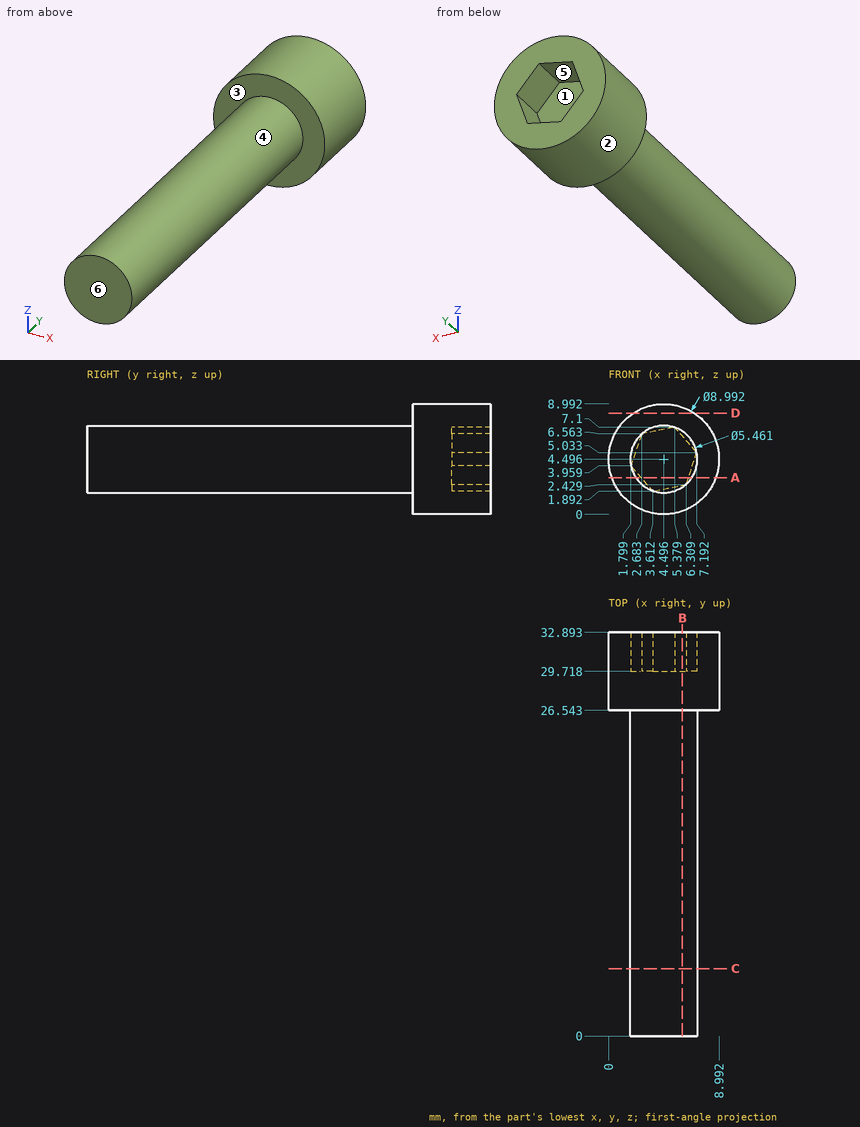
The drawing under review shows one solid part. Ordinate dimensions are in mm from its lowest x, y, z. A direction names the side the tool comes from. Coordinates: 2 decimals unless noted, no trailing zeros. Loops run counter-clockwise (first coordinate to the right, second up) from the corner with the lowest first, then second, coordinate; pieces in that order, holes last. Notation, with made-up numbers: (48, 7) -> (60, 7) arc R14 ccw to (60, 21) -> close; hole circle Ø10 at (63.25, 57). An arc over 180 degrees is marked (long way). Answer as a JSON object with one key per item and string values.
Q1. Clearance check with flat-ended pins moving along their axes: pin 1 Ø1 at (x, y) = (6.5, 8) entering from -Z; pin 2 Ø2 at (x, y) = (6.5, 6) entering from -Z; pin 3 Ø1 at (y, z) = (24.5, 3) entering from +X. State where each tip first meets the part, or that it passes through.
Answer block:
{"pin 1": "stops at z = 2.22", "pin 2": "stops at z = 1.96", "pin 3": "stops at x = 7.04"}
Q2. Take a section at D-D on z = 8.25. Give the boundary of the cut face in (x, y).
Answer block:
{"outline": "(2.02, 26.54) -> (6.97, 26.54) -> (6.97, 32.89) -> (2.02, 32.89) -> close"}
Q3. Take a section at B-B on x = 6. Give the boundary of the cut face in (y, z) (1 decimal).
Answer block:
{"outline": "(0, 2.2) -> (26.5, 2.2) -> (26.5, 0.3) -> (32.9, 0.3) -> (32.9, 2.4) -> (29.7, 2.4) -> (29.7, 6.4) -> (32.9, 6.4) -> (32.9, 8.7) -> (26.5, 8.7) -> (26.5, 6.8) -> (0, 6.8) -> close"}
Q4. Tool access review of the marked faces 1, 2 and 3: name each direction out of +Z, -Z, +X, -X, +Y, -Y from which nothing blocks a thin tool from reaching the whole face with its end or side.
Answer block:
{"face 1": "+Y", "face 2": "+Y, -Y", "face 3": "-Y"}
Q5. Take a section at A-A on z = 3. Give the boundary of the cut face in (x, y) (1 decimal).
Answer block:
{"outline": "(0.3, 26.5) -> (2.2, 26.5) -> (2.2, 0) -> (6.8, 0) -> (6.8, 26.5) -> (8.7, 26.5) -> (8.7, 32.9) -> (6.5, 32.9) -> (6.5, 29.7) -> (2.6, 29.7) -> (2.6, 32.9) -> (0.3, 32.9) -> close"}
Q6. The part is to be moulded in two halves that separate along Z. For the marked faces 4, 5 and 6, say which applies: +Z half, -Z half, draft (parallel to the pull), parting line (faces both ways), or undercut.
Answer block:
{"face 4": "parting line", "face 5": "undercut", "face 6": "draft"}
Q7. To check wall thickness, follow L1, parallel to Y at x = 7.75, z = 5.5; L2, parallel to Y at x = 4.5, z = 2.5; L3, parallel to X at y = 30.5, z = 3.5 (1 decimal). State the ranges of each line that lie inside material, in increasing order.
Answer block:
{"L1": "y = 26.54 to 32.89", "L2": "y = 0 to 29.72", "L3": "x = 0.1 to 2.2, 6.7 to 8.9"}
Q8. Take a section at C-C on y = 5.5. Give the boundary of the cut face in (x, z) (1 decimal), plus the area to 3 significant figures.
Answer block:
{"outline": "circle Ø5.5 at (4.5, 4.5)", "area": "23.4 mm^2"}
